```python
from build123d import *

# Parameters (mm, degrees)
SKETCH_1_R      = 2.0999999
EXTRUDE_1_DEPTH = 640


with BuildPart() as part:
    # 草圖1 → 填料-伸長1 (new body)
    with BuildSketch(Plane.XY):
        with BuildLine():
            Line((-10, 16.7), (-10, 3.3))
            ThreePointArc((-10, 3.3), (-9.912132034, 3.087867966), (-9.7, 3))
            Line((-9.7, 3), (-8, 3))
            Line((-8, 3), (-8, 6))
            Line((-8, 6), (-7.060650687, 6))
            Line((-7.060650687, 6), (-4, 2.939349))
            Line((-4, 2.939349), (-4, 0.519615242))
            Line((-4, 0.519615242), (-3.7, 0))
            Line((-3.7, 0), (-4, -0.519615242))
            Line((-4, -0.519615242), (-4, -2.9393502))
            Line((-4, -2.9393502), (-7.060649487, -6))
            Line((-7.060649487, -6), (-8, -6))
            Line((-8, -6), (-8, -3))
            Line((-8, -3), (-9.7, -3))
            ThreePointArc((-9.7, -3), (-9.912132034, -3.087867966), (-10, -3.3))
            Line((-10, -3.3), (-10, -16.7))
            ThreePointArc((-10, -16.7), (-9.912132034, -16.912132034), (-9.7, -17))
            Line((-9.7, -17), (-8, -17))
            Line((-8, -17), (-8, -14))
            Line((-8, -14), (-7.060672887, -14))
            Line((-7.060672887, -14), (-4, -17.0606732))
            Line((-4, -17.0606732), (-4, -19.480384758))
            Line((-4, -19.480384758), (-3.7, -20))
            Line((-3.7, -20), (-4, -20.519615242))
            Line((-4, -20.519615242), (-4, -22.93935665))
            Line((-4, -22.93935665), (-7.060643037, -26))
            Line((-7.060643037, -26), (-8, -26))
            Line((-8, -26), (-8, -23))
            Line((-8, -23), (-9.7, -23))
            ThreePointArc((-9.7, -23), (-9.912132034, -23.087867966), (-10, -23.3))
            Line((-10, -23.3), (-10, -29))
            ThreePointArc((-10, -29), (-9.707106781, -29.707106781), (-9, -30))
            Line((-9, -30), (-3.3, -30))
            ThreePointArc((-3.3, -30), (-3.087867966, -29.912132034), (-3, -29.7))
            Line((-3, -29.7), (-3, -28))
            Line((-3, -28), (-6, -28))
            Line((-6, -28), (-6, -27.060683408))
            Line((-6, -27.060683408), (-2.939316, -24))
            Line((-2.939316, -24), (-0.519095055, -24))
            Line((-0.519095055, -24), (1e-06, -23.7))
            Line((1e-06, -23.7), (0.518577868, -24))
            Line((0.518577868, -24), (2.939318, -24))
            Line((2.939318, -24), (6, -27.060682403))
            Line((6, -27.060682403), (6, -28))
            Line((6, -28), (3, -28))
            Line((3, -28), (3, -29.7))
            ThreePointArc((3, -29.7), (3.087867966, -29.912132034), (3.3, -30))
            Line((3.3, -30), (9, -30))
            ThreePointArc((9, -30), (9.707106781, -29.707106781), (10, -29))
            Line((10, -29), (10, -23.3))
            ThreePointArc((10, -23.3), (9.912132034, -23.087867966), (9.7, -23))
            Line((9.7, -23), (8, -23))
            Line((8, -23), (8, -26))
            Line((8, -26), (7.060637687, -26))
            Line((7.060637687, -26), (4, -22.93935641))
            Line((4, -22.93935641), (4, -20.519623992))
            Line((4, -20.519623992), (3.7, -20.00000875))
            Line((3.7, -20.00000875), (4, -19.480393508))
            Line((4, -19.480393508), (4, -17.06066109))
            Line((4, -17.06066109), (7.060655187, -14))
            Line((7.060655187, -14), (8, -14))
            Line((8, -14), (8, -17))
            Line((8, -17), (9.7, -17))
            ThreePointArc((9.7, -17), (9.912132034, -16.912132034), (10, -16.7))
            Line((10, -16.7), (10, -3.3))
            ThreePointArc((10, -3.3), (9.912132034, -3.087867966), (9.7, -3))
            Line((9.7, -3), (8, -3))
            Line((8, -3), (8, -6))
            Line((8, -6), (7.060651537, -6))
            Line((7.060651537, -6), (4, -2.93934815))
            Line((4, -2.93934815), (4, -0.519623992))
            Line((4, -0.519623992), (3.7, -8.75e-06))
            Line((3.7, -8.75e-06), (4, 0.519606492))
            Line((4, 0.519606492), (4, 2.9393426))
            Line((4, 2.9393426), (7.060657087, 6))
            Line((7.060657087, 6), (8, 6))
            Line((8, 6), (8, 3))
            Line((8, 3), (9.7, 3))
            ThreePointArc((9.7, 3), (9.912132034, 3.087867966), (10, 3.3))
            Line((10, 3.3), (10, 16.7))
            ThreePointArc((10, 16.7), (9.912132034, 16.912132034), (9.7, 17))
            Line((9.7, 17), (8, 17))
            Line((8, 17), (8, 14))
            Line((8, 14), (7.06065821, 14))
            Line((7.06065821, 14), (4, 17.060658523))
            Line((4, 17.060658523), (4, 19.480376008))
            Line((4, 19.480376008), (3.7, 19.99999125))
            Line((3.7, 19.99999125), (4, 20.519606492))
            Line((4, 20.519606492), (4, 22.939362173))
            Line((4, 22.939362173), (7.060637514, 26))
            Line((7.060637514, 26), (8, 26))
            Line((8, 26), (8, 23))
            Line((8, 23), (9.7, 23))
            ThreePointArc((9.7, 23), (9.912132034, 23.087867966), (10, 23.3))
            Line((10, 23.3), (10, 29))
            ThreePointArc((10, 29), (9.707106781, 29.707106781), (9, 30))
            Line((9, 30), (3.3, 30))
            ThreePointArc((3.3, 30), (3.087867966, 29.912132034), (3, 29.7))
            Line((3, 29.7), (3, 28))
            Line((3, 28), (6, 28))
            Line((6, 28), (6, 27.060684313))
            Line((6, 27.060684313), (2.939316, 24))
            Line((2.939316, 24), (0.519614242, 24))
            Line((0.519614242, 24), (-1e-06, 23.7))
            Line((-1e-06, 23.7), (-0.519616242, 24))
            Line((-0.519616242, 24), (-2.939318, 24))
            Line((-2.939318, 24), (-6, 27.060682313))
            Line((-6, 27.060682313), (-6, 28))
            Line((-6, 28), (-3, 28))
            Line((-3, 28), (-3, 29.7))
            ThreePointArc((-3, 29.7), (-3.087867966, 29.912132034), (-3.3, 30))
            Line((-3.3, 30), (-9, 30))
            ThreePointArc((-9, 30), (-9.707106781, 29.707106781), (-10, 29))
            Line((-10, 29), (-10, 23.3))
            ThreePointArc((-10, 23.3), (-9.912132034, 23.087867966), (-9.7, 23))
            Line((-9.7, 23), (-8, 23))
            Line((-8, 23), (-8, 26))
            Line((-8, 26), (-7.060644014, 26))
            Line((-7.060644014, 26), (-4, 22.939355673))
            Line((-4, 22.939355673), (-4, 20.519615242))
            Line((-4, 20.519615242), (-3.7, 20))
            Line((-3.7, 20), (-4, 19.480384758))
            Line((-4, 19.480384758), (-4, 17.060669373))
            Line((-4, 17.060669373), (-7.06066906, 14))
            Line((-7.06066906, 14), (-8, 14))
            Line((-8, 14), (-8, 17))
            Line((-8, 17), (-9.7, 17))
            ThreePointArc((-9.7, 17), (-9.912132034, 16.912132034), (-10, 16.7))
        make_face()
        with Locations((0, 20.000013123)):
            Circle(SKETCH_1_R, mode=Mode.SUBTRACT)
        Circle(SKETCH_1_R, mode=Mode.SUBTRACT)
        with Locations((0, -20.000013525)):
            Circle(SKETCH_1_R, mode=Mode.SUBTRACT)
        with BuildLine():
            Line((-7.7, 8), (-7.063594325, 8))
            ThreePointArc((-7.063594325, 8), (-6.948789288, 7.977163857), (-6.85146228, 7.912132024))
            Line((-6.85146228, 7.912132024), (-2.939330656, 4))
            Line((-2.939330656, 4), (2.939337056, 4))
            Line((2.939337056, 4), (6.85146868, 7.912132024))
            ThreePointArc((6.85146868, 7.912132024), (6.948795688, 7.977163857), (7.063600725, 8))
            Line((7.063600725, 8), (7.7, 8))
            ThreePointArc((7.7, 8), (7.912132034, 8.087867966), (8, 8.3))
            Line((8, 8.3), (8, 11.7))
            ThreePointArc((8, 11.7), (7.912132034, 11.912132034), (7.7, 12))
            Line((7.7, 12), (7.063601848, 12))
            ThreePointArc((7.063601848, 12), (6.948796811, 12.022836143), (6.851469803, 12.087867976))
            Line((6.851469803, 12.087867976), (2.939338179, 16))
            Line((2.939338179, 16), (-2.939349029, 16))
            Line((-2.939349029, 16), (-6.851480653, 12.087867976))
            ThreePointArc((-6.851480653, 12.087867976), (-6.948807661, 12.022836143), (-7.063612698, 12))
            Line((-7.063612698, 12), (-7.7, 12))
            ThreePointArc((-7.7, 12), (-7.912132034, 11.912132034), (-8, 11.7))
            Line((-8, 11.7), (-8, 8.3))
            ThreePointArc((-8, 8.3), (-7.912132034, 8.087867966), (-7.7, 8))
        make_face(mode=Mode.SUBTRACT)
        with BuildLine():
            Line((-8, -8.3), (-8, -11.7))
            ThreePointArc((-8, -11.7), (-7.912132034, -11.912132034), (-7.7, -12))
            Line((-7.7, -12), (-7.063616525, -12))
            ThreePointArc((-7.063616525, -12), (-6.948811488, -12.022836143), (-6.85148448, -12.087867976))
            Line((-6.85148448, -12.087867976), (-2.939352856, -16))
            Line((-2.939352856, -16), (2.939340746, -16))
            Line((2.939340746, -16), (6.851465031, -12.08786817))
            ThreePointArc((6.851465031, -12.08786817), (6.948792107, -12.022836196), (7.06359727, -12))
            Line((7.06359727, -12), (7.7, -12))
            ThreePointArc((7.7, -12), (7.912132034, -11.912132034), (8, -11.7))
            Line((8, -11.7), (8, -8.3))
            ThreePointArc((8, -8.3), (7.912132034, -8.087867966), (7.7, -8))
            Line((7.7, -8), (7.063595175, -8))
            ThreePointArc((7.063595175, -8), (6.948790138, -7.977163857), (6.85146313, -7.912132024))
            Line((6.85146313, -7.912132024), (2.939331506, -4))
            Line((2.939331506, -4), (-2.939329456, -4))
            Line((-2.939329456, -4), (-6.85146108, -7.912132024))
            ThreePointArc((-6.85146108, -7.912132024), (-6.948788088, -7.977163857), (-7.063593125, -8))
            Line((-7.063593125, -8), (-7.7, -8))
            ThreePointArc((-7.7, -8), (-7.912132034, -8.087867966), (-8, -8.3))
        make_face(mode=Mode.SUBTRACT)
    extrude(amount=-EXTRUDE_1_DEPTH)


solid = part.part
```
Geometry: final body of the model. Coordinates: model frame, mm. Coordinates: 2 decimals unless noted, no trailing zeros. Answer as CSV lines item,"result".
Q1. Line query: probe 1 along Y at (x, z) = (-7, -409.5); probe 2 along Y at (x, z) = (-2.5, -156); probe 3 along Y at (x, z) = (1.5, -31.5). Output: solid intervals per line, ascending. Write a range as [from, to].
Answers:
probe 1,"y = [-30, -25.94], [-14.06, -12.01], [-7.99, -5.94], [5.94, 7.99], [12.01, 14.06], [25.94, 30]"
probe 2,"y = [-24, -16], [-4, 4], [16, 24]"
probe 3,"y = [-24, -21.47], [-18.53, -16], [-4, -1.47], [1.47, 4], [16, 18.53], [21.47, 24]"
Q2. Section A-A on z = -286.5. Count the separate pieces of the cut face and the enclosed holes in it, and give its area (3 significant figures).
Answers:
separate pieces,"1"
enclosed holes,"5"
area,"465 mm^2"
Q3. First-contact query: P1, Ø3, axis at x = -1, z = -173.5, coming from the -Y side; P2, Ø3, axis at x = 1, z = -419, coming from the +Y side. Flat tips, straight axial feed; report the tip coordinate or a pass-through.
Answers:
P1,"stops at y = -24"
P2,"stops at y = 24"
